Geometry: final body of the model. Coordinates: model frame, mm. Face numbers are marked on the shaded views. Give positions to 0.01 mm unless a question says otherwise; leave off trailing zeros. Loops run counter-clockwise (first coordinate to the right, second up) from the corner with the lowest first, then second, coordinate; pieces in that order, holes last.
1. Section A-A, the plane x = 65. Output: boundary loops of the cut face in (y, z).
2. First-contact query: P1, Ø2.5, axis at x = 56.29, z = -32.5, coming from the +Y side (3 decimals); P2, Ø4, axis at y = 27.82, z = 0, coming from the -X side; P3, Ø4, axis at y = 31.5, z = -32, coming from the +X side; P4, Ø6, axis at y = 11.5, z = -16, coming from the -X side. Flat tips, straight axial feed; report the tip coordinate or a pass-through.
3. Material intervals for line 1 along Y through (x, z) = (0, 52.1); line 2 along Y through (x, z) = (63, -36); line 3 along Z through (x, y) = (0, 6), sorted ascending.
4. Draft query along Z for the marked faces 1, 2 and 3. Return one class per face: +Z half, -Z half, draft (parallel to the pull), parting line (faces both ways), or undercut.
from build123d import *

# Parameters (mm, degrees)
SKETCH5_R               = 55
SKETCH5_R_2             = 50.25
BOSS_EXTRUDE1_DEPTH     = 50
CUT_EXTRUDE1_DEPTH      = 211
CUT_EXTRUDE1_DEPTH_BACK = 106
SKETCH8_R               = 1.5
CUT_EXTRUDE2_DEPTH      = 93.466210222
CUT_EXTRUDE2_DEPTH_BACK = 93.466210222
SKETCH9_R               = 1.5
SKETCH14_R              = 75
SKETCH14_R_2            = 50.25
BOSS_EXTRUDE4_DEPTH     = 15
FILLET3_R               = 2.5
SKETCH15_R              = 1.5
CUT_EXTRUDE3_DEPTH      = 125.398553098
CIRPATTERN1_COUNT       = 6


with BuildPart() as part:
    # Sketch5 → Boss-Extrude1 (new body)
    with BuildSketch(Plane(origin=(0, 0, 0), x_dir=(1, 0, 0), z_dir=(0, 1, 0))):
        with Locations(Location((0, 0, 0), (0, 0, 270))):
            Circle(SKETCH5_R)
        with Locations(Location((0, 0, 0), (0, 0, 270))):
            Circle(SKETCH5_R_2, mode=Mode.SUBTRACT)
    extrude(amount=BOSS_EXTRUDE1_DEPTH)

    # Sketch8 → Cut-Extrude1 (cut, two sides: drawn at the far end of the back side and taken through both)
    with BuildSketch(Plane(origin=(0, 0, 0), x_dir=(0, 0, -1), z_dir=(1, 0, 0)).offset(-CUT_EXTRUDE1_DEPTH_BACK)):
        with Locations(Location((0, 27.82, 0), (0, 0, 180))):
            Circle(SKETCH8_R)
    extrude(amount=CUT_EXTRUDE1_DEPTH + CUT_EXTRUDE1_DEPTH_BACK, mode=Mode.SUBTRACT)

    # Sketch9 → Cut-Extrude2 (cut, two sides: drawn at the far end of the back side and taken through both)
    with BuildSketch(Plane.XY.offset(-CUT_EXTRUDE2_DEPTH_BACK)):
        with Locations((0, 27.82)):
            Circle(SKETCH9_R)
    extrude(amount=CUT_EXTRUDE2_DEPTH + CUT_EXTRUDE2_DEPTH_BACK, mode=Mode.SUBTRACT)

    # Sketch14 → Boss-Extrude4 (add)
    with BuildSketch(Plane(origin=(0, -15, 0), x_dir=(1, 0, 0), z_dir=(0, 1, 0))):
        with Locations(Location((0, 0, 0), (0, 0, 270))):
            Circle(SKETCH14_R)
        with Locations(Location((0, 0, 0), (0, 0, 270))):
            Circle(SKETCH14_R_2, mode=Mode.SUBTRACT)
    extrude(amount=BOSS_EXTRUDE4_DEPTH)

    # Fillet3
    fillet3_edges = [part.edges().sort_by_distance(p)[0] for p in [
        (0, 0, -55),
    ]]
    fillet(fillet3_edges, radius=FILLET3_R)

    # Sketch15 → Cut-Extrude3 (cut, through all)
    with BuildSketch(Plane.XZ.offset(15)):
        with Locations(Location((0, 65, 0), (0, 0, 270))):
            Circle(SKETCH15_R)
    cut_extrude3 = extrude(amount=-CUT_EXTRUDE3_DEPTH, mode=Mode.SUBTRACT)

    # CirPattern1: Cut-Extrude3 ×6 about axis
    cirpattern1_axis = Axis((0, 0, 0), (0, 1, 0))
    for i in range(1, CIRPATTERN1_COUNT):
        add(cut_extrude3.rotate(cirpattern1_axis, i * 360 / CIRPATTERN1_COUNT), mode=Mode.SUBTRACT)


solid = part.part
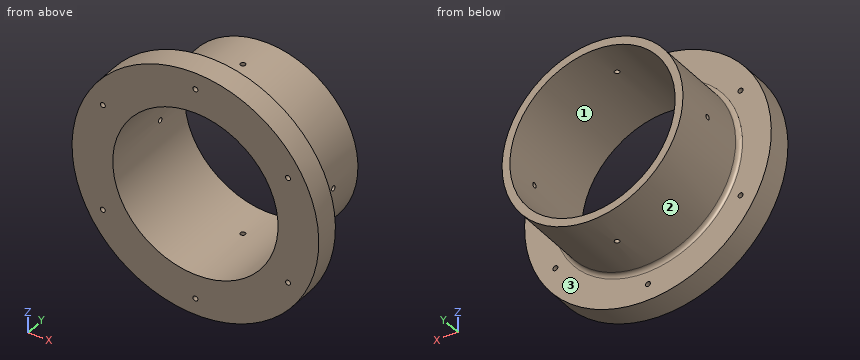
Answers below:
1. outline: (-15, -37.42) - (0, -37.42) - (0, 37.42) - (-15, 37.42) - close
2. P1: passes through
2. P2: stops at x = -55
2. P3: stops at x = 46.1
2. P4: stops at x = -53.44
3. line 1: y = -15 to 26.32, 29.32 to 50
3. line 2: y = -15 to 0
3. line 3: z = -55 to -50.25, 50.25 to 55
4. face 1: undercut
4. face 2: parting line
4. face 3: draft
